from build123d import *

# Parameters (mm, degrees)
FILLET1_R          = 1.27
SKETCH2_R          = 2.667
CUT_EXTRUDE1_DEPTH = 3.81
CIRPATTERN1_COUNT  = 12
FILLET2_R          = 0.254


with BuildPart() as part:
    # Chamber Revolve → Revolve1 (revolve)
    with BuildSketch(Plane.XY):
        Polygon((3.81, 22.86), (61.331753256, 22.86), (61.331753256, 11.43), (43.197991731, 7.57555), (41.673991731, 7.57555), (38.1, 15.24), (0, 15.24), (0, 19.304), (1.016, 19.304), (1.016, 21.844), (0, 21.844), (0, 33.02), (3.81, 33.02), align=None)
    revolve(axis=Axis((0, 0, 0), (1, 0, 0)))

    # Fillet1
    fillet1_edges = [part.edges().sort_by_distance(p)[0] for p in [
        (3.81, -22.86, 0),
    ]]
    fillet(fillet1_edges, radius=FILLET1_R)

    # Sketch2 → Cut-Extrude1 (cut)
    with BuildSketch(Plane.ZY):
        with Locations((0, 27.94)):
            Circle(SKETCH2_R)
    cut_extrude1 = extrude(amount=-CUT_EXTRUDE1_DEPTH, mode=Mode.SUBTRACT)

    # CirPattern1: Cut-Extrude1 ×12 about axis
    cirpattern1_axis = Axis((0, 0, 0), (1, 0, 0))
    for i in range(1, CIRPATTERN1_COUNT):
        add(cut_extrude1.rotate(cirpattern1_axis, i * 360 / CIRPATTERN1_COUNT), mode=Mode.SUBTRACT)

    # Fillet2
    fillet2_edges = [part.edges().sort_by_distance(p)[0] for p in [
        (1.016, -19.304, 0),
        (1.016, -21.844, 0),
    ]]
    fillet(fillet2_edges, radius=FILLET2_R)


solid = part.part
Geometry check sheet. Reference: the model listing, model coordinates, mm. A direction names the side the tool comes from. Round coordinates to 2 decimals unless told otherwise and drop trailing zeros. Loops run counter-clockwise (first coordinate to the right, second up) from the corner with the lowest first, then second, coordinate; pieces in that order, holes last. Notation, with made-up numbers: (-8.75, 58) - (42.25, 58) arc R23 ccw to (42.25, 81) - close; hole circle Ø9 at (17.25, 84.5). An arc over 180 degrees is marked (long way). Answer as CSV lines item,"result".
(1) Cross-section at A-A, the plane y = 27.94. Enter the section's corners in (x, z), and give its area (3 significant figures).
Output values:
outline,"(0, -17.6) - (3.81, -17.6) - (3.81, -2.67) - (0, -2.67) - close; (0, 2.67) - (3.81, 2.67) - (3.81, 17.6) - (0, 17.6) - close"
area,"114 mm²"
(2) Depth check by flat-ended pin: pin 1 Ø6 at (y, z) = (-27.94, 0) entering from +X; pin 2 Ø24 at (y, z) = (0, 0) entering from -X; pin 3 Ø5 at (y, z) = (-24.2, 13.97) entering from +X; pin 4 Ø10 at (x, y) = (50, -13) entering from +Z. Enter the tip coordinate at first touch or a pass-through.
Output values:
pin 1,"stops at x = 3.81"
pin 2,"stops at x = 39.61"
pin 3,"passes through"
pin 4,"stops at z = 21.41"
(3) Cross-section at D-D, the plane z = 0. Give the number of separate pieces and of enclosed holes in the cut face, and give its area (3 significant figures).
Output values:
separate pieces,"4"
enclosed holes,"0"
area,"1,230 mm²"
(4) Set-up check for faces 5 (the face through (1.878, 26.162, -12.168)), 6 (the face through (18.78, -3.3, -14.88)): record each of +Z, -Z, +X, -X, +Y, -Y from which the full face is reachable in a straight line by a thin tool's end or side.
Output values:
face 5,"+X, -X"
face 6,"-X"
(5) Cross-section at C-C, the plane z = -29. Enter the section's corners in (x, y), and give its area (3 significant figures).
Output values:
outline,"(0, -15.79) - (3.81, -15.79) - (3.81, -2.45) - (0, -2.45) - close; (0, 2.45) - (3.81, 2.45) - (3.81, 15.79) - (0, 15.79) - close"
area,"102 mm²"
(6) Material ranges on line 1 along Z through (x, y) = (12, 0); line 2 along X through (y, z) = (19, 4.5); line 3 along X through (y, z) = (29, -7), recorded low to high.
Output values:
line 1,"z = -22.86 to -15.24, 15.24 to 22.86"
line 2,"x = 1.01 to 61.33"
line 3,"x = 0 to 3.81"
(7) Release check for a two-part mould opening along Y. For faces 1 (the face through (1.878, -12.168, -26.162)), 2 (the face through (3.81, -9.9, 22.2)), 3 (the face through (1.9, 31.5, 9.9)), 4 (the face through (1.878, -25.427, -16.336)) record: released by +Y, released by -Y, zero draft, split by the parting line, or undercut.
Output values:
face 1,"undercut"
face 2,"zero draft"
face 3,"split by the parting line"
face 4,"undercut"
(8) Cross-section at B-B, the plane x = 6.5. Enter the section's corners in (y, z).
Output values:
outline,"circle Ø45.72 at (0, 0); hole circle Ø30.48 at (0, 0)"
